Read the model definition and answer for the solid it produces. Units are mm, in the model's axes. A direction names the side the tool comes from. Give positions to 0.01 mm unless a question says otherwise; leave off trailing zeros. Order: outer loops, then holes, each group sorted by start corner. A loop starts at its lowest first (then second) coordinate and runs counter-clockwise, first axis right, second up. Notation, with made-up numbers: M -28,-28.5 L 0,-28.5 A11 ccw 0,-23.5 Z; hole C 83.5,34.25 d7. An arc over 180 degrees is marked long. One line per item, written item: value.
from build123d import *

# Parameters (mm, degrees)
ESQUISSE1_R             = 30
BASE_EXTRUSION_DEPTH    = 900
COQUE1_T                = -2.5
ENL_V_MAT_EXTRU_1_DEPTH = 100
ESQUISSE4_W             = 89
ESQUISSE4_H             = 20
BOSS_EXTRU_1_DEPTH      = 2
ESQUISSE3_R             = 6
ENL_V_MAT_EXTRU_2_DEPTH = 100
ESQUISSE6_R             = 3
ENL_V_MAT_EXTRU_3_DEPTH = 50


with BuildPart() as part:
    # Esquisse1 → Base-Extrusion (new body)
    with BuildSketch(Plane(origin=(0, 0, 0), x_dir=(0, 0, -1), z_dir=(1, 0, 0))):
        with Locations(Location((0, 0, 0), (0, 0, 140.05549481))):
            Circle(ESQUISSE1_R)
    extrude(amount=BASE_EXTRUSION_DEPTH)

    # Coque1
    coque1_openings = [part.faces().sort_by_distance(p)[0] for p in [
        (0, 0, 0),
        (900, 0, 0),
    ]]
    offset(amount=COQUE1_T, openings=coque1_openings, kind=Kind.INTERSECTION)

    # Esquisse2 → Enlèv. mat.-Extru.1 (cut)
    with BuildSketch(Plane(origin=(0, 0, 0), x_dir=(1, 0, 0), z_dir=(0, 1, 0))):
        with BuildLine():
            Line((-10, 23), (48, 23))
            ThreePointArc((48, 23), (63.556349186, 16.556349186), (70, 1))
            Line((70, 1), (70, -1))
            ThreePointArc((70, -1), (63.556349186, -16.556349186), (48, -23))
            Line((48, -23), (-10, -23))
            Line((-10, -23), (-10, 23))
        make_face()
    extrude(amount=ENL_V_MAT_EXTRU_1_DEPTH, mode=Mode.SUBTRACT)

    # Esquisse4 → Boss.-Extru.1 (add)
    with BuildSketch(Plane(origin=(0, 26, 0), x_dir=(-1, 0, 0), z_dir=(0, 1, 0))):
        with Locations((-115.5, 0)):
            Rectangle(ESQUISSE4_W, ESQUISSE4_H)
    extrude(amount=BOSS_EXTRU_1_DEPTH)

    # Esquisse3 → Enlèv. mat.-Extru.2 (cut)
    with BuildSketch(Plane(origin=(0, 0, 0), x_dir=(1, 0, 0), z_dir=(0, 1, 0))):
        with Locations(Location((85, 0, 0), (0, 0, 90))):
            Circle(ESQUISSE3_R)
        with Locations(Location((145, 0, 0), (0, 0, 90))):
            Circle(ESQUISSE3_R)
    extrude(amount=ENL_V_MAT_EXTRU_2_DEPTH, mode=Mode.SUBTRACT)

    # Esquisse6 → Enlèv. mat.-Extru.3 (cut)
    with BuildSketch(Plane.XY):
        with Locations((880, 0)):
            Circle(ESQUISSE6_R)
    extrude(amount=-ENL_V_MAT_EXTRU_3_DEPTH, mode=Mode.SUBTRACT)


solid = part.part
1) Consider probe 1 along X at (y, z) = (27.45, 0); probe 2 along Z at (x, y) = (687, 0). Determine where each line is inside the solid, lowest interval first.
Reported:
probe 1: x = 71 to 79, 91 to 139, 151 to 160
probe 2: z = -30 to -27.5, 27.5 to 30
2) Each of these flat-tipped pins is pushed along its axis until it touches: pin 1 Ø4 at (y, z) = (23, 11.5) entering from -X; pin 2 Ø4.5 at (x, y) = (35, 17) entering from -Z; pin 3 Ø4 at (x, y) = (802, -18.5) entering from -Z. Where does it stop, or does it pass through?
Reported:
pin 1: stops at x = 66.36
pin 2: stops at z = -26.12
pin 3: stops at z = -25.05
3) Determine the mould class of faces 4 (the face through (0, -28, 5)), 5 (the face through (443.7, -27.263, -3.606)), 6 (the face through (443.7, -29.74, -3.93)) for opening direction Y: +Y half, -Y half, draft (parallel to the pull), parting line (faces both ways), or undercut.
Reported:
face 4: draft
face 5: undercut
face 6: parting line
4) Find section A-A, the plane y = -14. Write down the section's boundary in (x, z), plus the area to 3 significant figures.
Reported:
outline: M 0,-26.53 L 900,-26.53 L 900,-23.67 L 0,-23.67 Z; M 0,23.67 L 900,23.67 L 900,26.53 L 0,26.53 Z
area: 5,150 mm^2
5) Which of the six approach directions +Z, -Z, +X, -X, +Y, -Y give full straight-line access (tool end or side, diameter ignored) to faces 1 (the face through (61.58, 21.94, -18.31)), 2 (the face through (116, 26, 0)), 3 (the face through (900, 27.1, -5.5))?
Reported:
face 1: -X, +Y
face 2: +X, -X
face 3: +Z, -Z, +X, +Y, -Y
6) Find section B-B, the plane x = 190.5. Write down the section's boundary in (y, z).
Reported:
outline: C 0,0 d60; hole C 0,0 d55
